The model under review builds one solid part; all positions refer to its coordinate system, in mm. Round coordinates to 2 decimals unless told otherwise and drop trailing zeros. Loops run counter-clockwise (first coordinate to the right, second up) from the corner with the lowest first, then second, coordinate; pieces in that order, holes last. Notation, with made-up numbers: M 10.25,25 L 30.25,25 A15 ccw 30.25,38 Z; hole C 18,45 d3. An arc over 180 degrees is marked long. Use a Markdown table: item, result. Add a question column.
```python
from build123d import *

# Parameters (mm, degrees)
F0_R     = 21.43125
F1_DEPTH = 254
F2_SIZE  = 1.524
F4_D     = 14.68374
F4_DEPTH = 38.1
F4_TIP   = 4.411440553
F6_W     = 7.112
F6_H     = 3.048
F7_DEPTH = 42.8635


with BuildPart() as f1:
    # F0 (on Right) → F1 (new body, symmetric)
    with BuildSketch(Plane.YZ):
        Circle(F0_R)
    extrude(amount=F1_DEPTH, both=True)

    # F2
    f2_edges = [f1.edges().sort_by_distance(p)[0] for p in [
        (254, -21.43125, 0),
        (-254, -21.43125, 0),
    ]]
    chamfer(f2_edges, length=F2_SIZE)

    # F4
    with Locations(Plane.YZ.offset(254)):
        with Locations((0, 0)):
            Hole(F4_D / 2, depth=F4_DEPTH)
            with Locations((0, 0, -(F4_DEPTH + F4_TIP / 2))):  # 118° drill point
                Cone(0, F4_D / 2, F4_TIP, mode=Mode.SUBTRACT)

    # F6 (on offset) → F7 (cut, through all)
    with BuildSketch(Plane.XZ.offset(21.43125)):
        with Locations((244.856, -19.90725)):
            Rectangle(F6_W, F6_H)
    extrude(amount=-F7_DEPTH, mode=Mode.SUBTRACT)


solid = f1.part
```
(1) To check wall thickness, follow probe 1 along Z at (x, y) = (176, -1.5); probe 2 along Y at (x, z) = (80.5, -1); probe 3 along Z at (x, y) = (86.5, -16). State the ranges of each line that lie inside material, in increasing order.
(2) Consider section A-A, the plane x = -178. Give the boundary of the cut face in (y, z), then the cut area to 3 significant figures.
(3) Draft analysis for pull direction Z (two halves, no side actions). For faces 1 (the face through (3.53, 11.52, 18.07)), 2 (the face through (212.255, -0.276, -1.245)), 3 (the face through (234.683, 1.592, -7.167)), 4 (the face through (-254, 0, 0)), state which applies: released by +Z, released by -Z, zero draft, split by the parting line, or undercut.
(4) Insertion check: pin 1 Ø8 at (x, z) = (42.5, -7.5) entering from -Y; pin 2 Ø8 at (x, y) = (-147, -17) entering from +Z; pin 3 Ø5.5 at (x, y) = (245, -2.5) entering from -Z. Each pin has a flat end and moves straight along its axis. Give the tip position at first contact, or say it passes through.
Found:
| question | item | result |
|---|---|---|
| 1 | probe 1 | z = -21.38 to 21.38 |
| 1 | probe 2 | y = -21.41 to 21.41 |
| 1 | probe 3 | z = -14.26 to 14.26 |
| 2 | outline | C 0,0 d42.86 |
| 2 | area | 1,440 mm^2 |
| 3 | face 1 | split by the parting line |
| 3 | face 2 | undercut |
| 3 | face 3 | undercut |
| 3 | face 4 | zero draft |
| 4 | pin 1 | stops at y = -21.14 |
| 4 | pin 2 | stops at z = 17.04 |
| 4 | pin 3 | stops at z = -18.38 |
